The listing builds one solid part. Answer for the finished solid, in the listing's coordinates (mm). Face numbers are marked on the shaded views. A direction names the side the tool comes from. Coordinates: 2 decimals unless noted, no trailing zeros. Order: outer loops, then holes, each group sorted by start corner. A loop starts at its lowest first (then second) coordinate and runs counter-clockwise, first axis right, second up. Notation, with made-up numbers: (77.25, 37) - (120.25, 37) arc R17 ccw to (120.25, 54) - close; hole circle Ø9 at (-36, -30). An arc over 180 degrees is marked (long way). One line per item, written item: value. Start each with the question number.
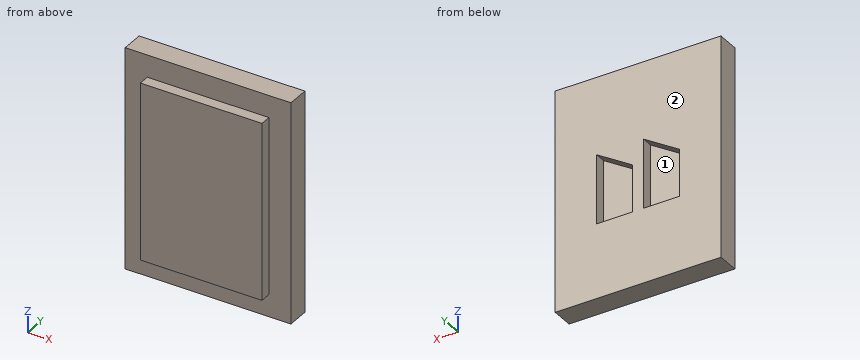
```python
from build123d import *

# Parameters (mm, degrees)
F0_W     = 12
F0_H     = 16
F0_W_2   = 8.8
F0_H_2   = 12.8
F1_DEPTH = 1.6
F2_DEPTH = 2.4
F3_DEPTH = 0.8


with BuildPart() as f1:
    # F0 (on Front) → F1 (new body)
    with BuildSketch(Plane.XZ):
        with Locations((-6, 8)):
            Rectangle(F0_W, F0_H)
        with Locations((-6, 8)):
            Rectangle(F0_W_2, F0_H_2, mode=Mode.SUBTRACT)
    extrude(amount=F1_DEPTH)

    # F0 (on Front) → F2 (join)
    with BuildSketch(Plane.XZ):
        with Locations((-6, 8)):
            Rectangle(F0_W_2, F0_H_2)
        Polygon((-9, 10.4), (-6.4, 10.4), (-6.4, 5.4), (-9, 5.4), (-9, 8.8), align=None, mode=Mode.SUBTRACT)
        Polygon((-5.6, 10.4), (-3, 10.4), (-3, 5.4), (-5.6, 5.4), (-5.6, 8.8), align=None, mode=Mode.SUBTRACT)
        Polygon((-3, 5.4), (-3, 10.4), (-5.6, 8.8), (-5.6, 5.4), align=None)
        Polygon((-5.6, 8.8), (-3, 10.4), (-5.6, 10.4), align=None)
        Polygon((-6.4, 5.4), (-6.4, 10.4), (-9, 8.8), (-9, 5.4), align=None)
        Polygon((-9, 8.8), (-6.4, 10.4), (-9, 10.4), align=None)
    extrude(amount=F2_DEPTH)

    # F0 (on Front) → F3 (cut)
    with BuildSketch(Plane.XZ):
        Polygon((-3, 5.4), (-3, 10.4), (-5.6, 8.8), (-5.6, 5.4), align=None)
        Polygon((-6.4, 5.4), (-6.4, 10.4), (-9, 8.8), (-9, 5.4), align=None)
    extrude(amount=F3_DEPTH, mode=Mode.SUBTRACT)


solid = f1.part
```
(1) For the marked faces 1 and 2, determine the directions among +Z, -Z, +X, -X, +Y, -Y from which every point of the face is accessible in a straight line to the end or side of a thin tool.
(2) The part is cut by section C-C on x = -9.25. Determine the outline of the cut face in (y, z), plus the area to 3 significant figures.
(3) The part is cut by section A-A on y = -0.5. Determine the outline of the cut face in (x, z), plus the area to 3 significant figures.
(4) Flat-ended cylindrical pins translate along their axes: pin 1 Ø0.8 at (x, z) = (-4, 8) entering from +Y; pin 2 Ø0.6 at (y, z) = (-2, 7) entering from -X. Find the tip coordinate at first contact, or state that the pin passes through.
(5) The part is cut by section B-B on z = 5.75. Determine the outline of the cut face in (x, y), plus the area to 3 significant figures.
(6) Consider probe 1 along X at (y, z) = (-1.75, 5.5); probe 2 along Y at (x, z) = (-10.5, 5); probe 3 along Z at (x, y) = (-8.5, -0.7). Determine where each line is inside the solid, lowest interval first.
(7) The part is cut by section D-D on z = 2.5. Determine the outline of the cut face in (x, y).
Completed:
1. face 1: +Y
1. face 2: +Z, -Z, +X, -X, +Y
2. outline: (-2.4, 1.6) - (-1.6, 1.6) - (-1.6, 0) - (0, 0) - (0, 16) - (-1.6, 16) - (-1.6, 14.4) - (-2.4, 14.4) - close
2. area: 35.8 mm2
3. outline: (-12, 0) - (0, 0) - (0, 16) - (-12, 16) - close; hole (-9, 5.4) - (-6.4, 5.4) - (-6.4, 10.4) - (-9, 8.8) - close; hole (-5.6, 5.4) - (-3, 5.4) - (-3, 10.4) - (-5.6, 8.8) - close
3. area: 170 mm2
4. pin 1: stops at y = -0.8
4. pin 2: stops at x = -10.4
5. outline: (-12, -1.6) - (-10.4, -1.6) - (-10.4, -2.4) - (-1.6, -2.4) - (-1.6, -1.6) - (0, -1.6) - (0, 0) - (-3, 0) - (-3, -0.8) - (-5.6, -0.8) - (-5.6, 0) - (-6.4, 0) - (-6.4, -0.8) - (-9, -0.8) - (-9, 0) - (-12, 0) - close
5. area: 22.1 mm2
6. probe 1: x = -10.4 to -1.6
6. probe 2: y = -1.6 to 0
6. probe 3: z = 0 to 5.4, 9.11 to 16
7. outline: (-12, -1.6) - (-10.4, -1.6) - (-10.4, -2.4) - (-1.6, -2.4) - (-1.6, -1.6) - (0, -1.6) - (0, 0) - (-12, 0) - close
